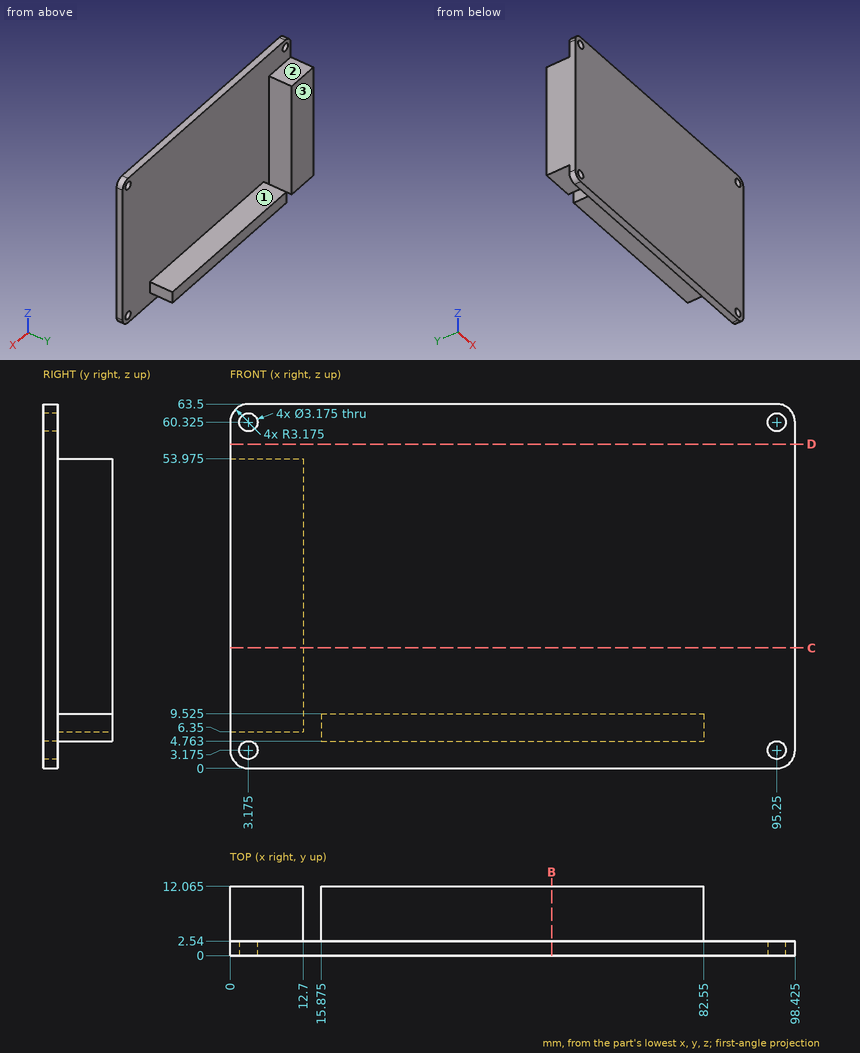
Verification items for this drawing (mm, ordinates from the low corner). A direction names the side the tool comes from. Round coordinates to 2 decimals unless told otherwise and drop trailing zeros. Write each loop counter-clockwise with the first axis right and the second up, starting at its lowest first coordinate (ties: lowest second). Pieces come first, ordered by that corner, then holes. Notation, with made-up numbers: M -17.5,-25.5 L 30.5,-25.5 A9 cw 30.5,-20.5 Z; hole C 2,-37.75 d10. An arc over 180 degrees is marked long. Write item = value, one per line. Start each with the question number.
1. Gauge pin test, flat ends, axial feed: pin 1 (2.5 mm diameter, centred on x = 95.25, z = 3.175, fed in from +Y); pin 2 (5 mm diameter, centred on x = 65, y = 7.5, fed in from -Z); pin 3 (5 mm diameter, centred on x = 5, y = 9, fed in from -Z); pin 4 (1.5 mm diameter, centred on x = 52, z = 34.5, fed in from -Y). Record the tip position at first contact, or that the pin passes through.
2. Section check C-C, the plane z = 21. Record the cut outline in (x, y) (1 decimal).
3. Tool access check on the marked faces 1, 2 and 3. Record the directions out of +Z, -Z, +X, -X, +Y, -Y that give a thin tool (end or side, any length) a straight path to the whole face; none if there is none.
4. Section check D-D, the plane z = 56.5. Record the cut outline in (x, y) (1 decimal), then the cut area to 3 significant figures.
5. Scan lines: line 1 (Z direction, x = 95.25, y = 1.45); line 2 (Y direction, x = 41, z = 13); line 3 (Z direction, x = 55, y = 11.75) (1 decimal). Record each from-to range of solid material in increasing order. Write a range as [from, to].
6. Section check B-B, the plane x = 56. Record the cut outline in (y, z) (1 decimal).
Results found:
q1.pin_1 = through
q1.pin_2 = 4.76
q1.pin_3 = 6.35
q1.pin_4 = 0
q2.outline = M 0,0 L 98.4,0 L 98.4,2.5 L 12.7,2.5 L 12.7,12.1 L 0,12.1 Z
q3.face_1 = +Z, +X, +Y
q3.face_2 = +Z, +X, -X, +Y
q3.face_3 = +Z, -Z, +X, -X, +Y
q4.outline = M 0,0 L 98.4,0 L 98.4,2.5 L 0,2.5 Z
q4.area = 250 mm^2
q5.line_1 = [0, 1.59], [4.76, 58.74], [61.91, 63.5]
q5.line_2 = [0, 2.54]
q5.line_3 = [4.8, 9.5]
q6.outline = M 0,0 L 2.5,0 L 2.5,4.8 L 12.1,4.8 L 12.1,9.5 L 2.5,9.5 L 2.5,63.5 L 0,63.5 Z
